Here's how the part is built. I have some questions about the finished solid (model axes, mm). Face numbers are marked on the shaded views. A direction names the side the tool comes from. Round coordinates to 2 decimals unless told otherwise and drop trailing zeros. Loops run counter-clockwise (first coordinate to the right, second up) from the corner with the lowest first, then second, coordinate; pieces in that order, holes last. Notation, with made-up numbers: M -8.5,78 L 23.5,78 A25 cw 23.5,90 Z; hole C 37.25,48 d10. An arc over 180 degrees is marked long. Answer as a JSON object with one key per item and string values.
from build123d import *

# Parameters (mm, degrees)
F0_W      = 60
F0_H      = 30
F1_DEPTH  = 30
F2_R      = 14.99999
F4_DEPTH  = 45.974
F5_DEPTH  = 11.5
F7_DEPTH  = 11.5
F8_R      = 7.5
F9_DEPTH  = 31
F11_DEPTH = 25.4
F13_DEPTH = 25.4


# Not quite as in the source:
# - a fillet or chamfer is up to 0.001 mm smaller than in the source, because OpenCascade refuses the exact size


with BuildPart() as f1:
    # F0 (on Front) → F1 (new body)
    with BuildSketch(Plane.XZ):
        with Locations((-1.155378297, 6.3267682405)):
            Rectangle(F0_W, F0_H)
    extrude(amount=F1_DEPTH)

    # F2 (radius 15 in the source; OpenCascade refuses exactly that, so slightly less here)
    f2_edges = [f1.edges().sort_by_distance(p)[0] for p in [
        (-31.155378, -15, 21.326768),
        (-31.155378, -15, -8.673232),
    ]]
    fillet(f2_edges, radius=F2_R)

    # F3 (on face) → F4 (cut)
    with BuildSketch(Plane.XY.offset(21.3267682405)):
        Polygon((28.844621703, 0), (1.844621703, 0), (28.844621703, -21), align=None)
    extrude(amount=-F4_DEPTH, mode=Mode.SUBTRACT)

    # F3 (on face) → F5 (cut)
    with BuildSketch(Plane.XY.offset(21.3267682405)):
        Polygon((28.844621703, -21), (1.844621703, 0), (1.844621703, -21), align=None)
    extrude(amount=-F5_DEPTH, mode=Mode.SUBTRACT)

    # F6 (on face) → F7 (cut)
    with BuildSketch(Plane(origin=(0, 0, -8.6732317595), x_dir=(1, 0, 0), z_dir=(0, 0, -1))):
        Polygon((1.844621703, 21), (1.844621703, 0), (28.844621703, 21), align=None)
    extrude(amount=-F7_DEPTH, mode=Mode.SUBTRACT)

    # F8 (on face) → F9 (cut)
    with BuildSketch(Plane(origin=(0, 0, 0), x_dir=(-1, 0, 0), z_dir=(0, 1, 0))):
        with Locations((16.155378297, 6.3267682405)):
            Circle(F8_R)
    extrude(amount=-F9_DEPTH, mode=Mode.SUBTRACT)

    # F10 (on face) → F11 (cut)
    with BuildSketch(Plane(origin=(0, -21, 0), x_dir=(-1, 0, 0), z_dir=(0, 1, 0))):
        Polygon((-28.844621703, 0.3183682405), (-28.844621703, -8.6732317595), (-19.844621703, -8.6732317595), align=None)
    extrude(amount=-F11_DEPTH, mode=Mode.SUBTRACT)

    # F12 (on face) → F13 (cut)
    with BuildSketch(Plane(origin=(0, -21, 0), x_dir=(-1, 0, 0), z_dir=(0, 1, 0))):
        Polygon((-19.853021703, 21.3267682405), (-28.844621703, 21.3267682405), (-28.844621703, 12.3267682405), align=None)
    extrude(amount=-F13_DEPTH, mode=Mode.SUBTRACT)


solid = f1.part
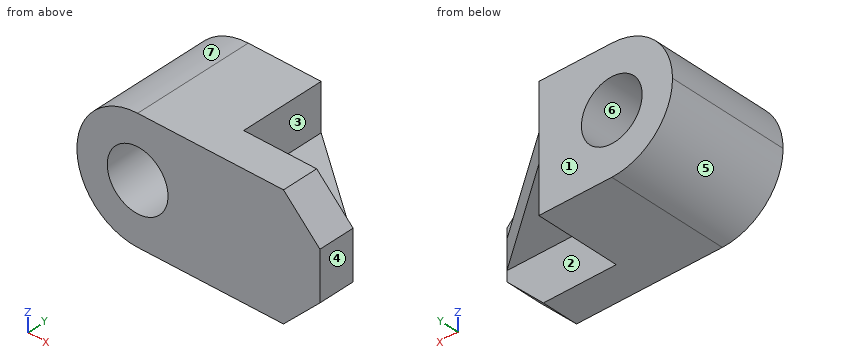
Item 1: I want a section at D-D on x = 9.5. List the corners of the cut face in (y, z) for me, plus the area to 3 significant figures.
Solution:
{"outline": "M -30,-8.67 L -21,-8.67 L -21,2.83 L -5.95,2.83 L -5.95,9.83 L -21,9.83 L -21,21.33 L -30,21.33 Z", "area": "375 mm2"}
Item 2: If I drill on L1, parallel to X at y = -26.5, z = 6.5; L2, parallel to Z at x = -16.5, y = -9; L3, parallel to Z at x = 16.5, y = -20, over which ranges is the centre line in solid material (lowest first)? Write a range as from..to.
Solution:
{"L1": "x = -31.15..-23.65, -8.66..28.84", "L2": "z = -8.67..-1.17, 13.82..21.32", "L3": "z = 2.83..9.83"}
Item 3: For P1, Ø6, axis at y = -11, z = 10, coming from the -X side; P2, Ø3.5, axis at x = 11.5, z = 18.5, coming from the +Y side; P3, Ø8, axis at x = -23.5, y = -21, coming from the -Z side, each with a flat end and sliding along its axis, tell me the tip position at first contact or that it passes through.
Solution:
{"P1": "stops at x = -31.14", "P2": "stops at y = -21", "P3": "stops at z = -8.3"}
Item 4: We'd pull the mould along Z, two halves only. Please class the marked faces 4, 5, 6 and 7: +Z half, -Z half, draft (parallel to the pull), parting line (faces both ways), or undercut.
Solution:
{"face 4": "draft", "face 5": "-Z half", "face 6": "undercut", "face 7": "+Z half"}
Item 5: I want a section at B-B on x = -20. List the corners of the cut face in (y, z) for me, plus the area to 3 significant figures.
Solution:
{"outline": "M -30,-8.17 L 0,-8.17 L 0,-0.11 L -30,-0.11 Z; M -30,12.77 L 0,12.77 L 0,20.83 L -30,20.83 Z", "area": "484 mm2"}
Item 6: I want a section at A-A on z = 5.5. List the corners of the cut face in (x, y) for me.
Solution:
{"outline": "M -31.13,-30 L -23.61,-30 L -23.61,0 L -31.13,0 Z; M -8.7,-30 L 28.84,-30 L 28.84,-21 L 1.84,0 L -8.7,0 Z"}
Item 7: For the marked faces 1, 2 and 3, which set-ups out of +Z, -Z, +X, -X, +Y, -Y let a thin tool reach every point of the face, with its end or its side?
Solution:
{"face 1": "+Z, -Z, +X, -X, +Y", "face 2": "-Z, +X, +Y", "face 3": "+Z, +X, +Y"}
